from build123d import *

# Parameters (mm, degrees)
BOSS_EXTRUDE1_DEPTH     = 7
SKETCH2_R               = 5
CUT_EXTRUDE1_DEPTH      = 7
LPATTERN1_COUNT         = 7
LPATTERN1_PITCH         = 30
SKETCH6_R               = 5
CUT_EXTRUDE2_DEPTH      = 10
BOSS_EXTRUDE2_DEPTH     = 21
CUT_EXTRUDE3_DEPTH      = 21
CUT_EXTRUDE4_REACH      = 220.014
SKETCH9_R               = 1.5
CUT_EXTRUDE5_REACH      = 220.771
SKETCH10_W              = 5.271518542
SKETCH10_H              = 23.219312301
BOSS_EXTRUDE3_DEPTH     = 14
CUT_EXTRUDE6_DEPTH      = 1
CUT_EXTRUDE6_DEPTH_BACK = 22
SKETCH12_W              = 22.7
SKETCH12_H              = 12.3
CUT_EXTRUDE7_DEPTH      = 7
CUT_EXTRUDE7_DEPTH_BACK = 7
SKETCH13_R              = 1
CUT_EXTRUDE8_REACH      = 184.393
SKETCH14_W              = 12
SKETCH14_H              = 10
CUT_EXTRUDE9_REACH      = 220.014
SKETCH15_R              = 2.5


with BuildPart() as part:
    # Sketch1 → Boss-Extrude1 (new body)
    with BuildSketch(Plane.XY):
        with BuildLine():
            Line((-200, 0), (50, 0))
            ThreePointArc((50, 0), (65, -15), (50, -30))
            Line((50, -30), (-200, -30))
            ThreePointArc((-200, -30), (-215, -15), (-200, 0))
        make_face()
    extrude(amount=BOSS_EXTRUDE1_DEPTH)

    # Sketch2 → Cut-Extrude1 (cut)
    with BuildSketch(Plane.XY.offset(7)):
        with Locations((-185, -15)):
            Circle(SKETCH2_R)
    cut_extrude1 = extrude(amount=-CUT_EXTRUDE1_DEPTH, mode=Mode.SUBTRACT)

    # LPattern1: Cut-Extrude1 ×7
    with Locations(*[(i * LPATTERN1_PITCH, 0, 0) for i in range(1, LPATTERN1_COUNT)]):
        add(cut_extrude1, mode=Mode.SUBTRACT)

    # Sketch6 → Cut-Extrude2 (cut)
    with BuildSketch(Plane(origin=(0, 0, 0), x_dir=(-1, 0, 0), z_dir=(0, 0, -1))):
        with Locations((-50, -15)):
            Circle(SKETCH6_R)
    extrude(amount=-CUT_EXTRUDE2_DEPTH, mode=Mode.SUBTRACT)

    # Sketch7 → Boss-Extrude2 (add)
    with BuildSketch(Plane(origin=(0, 0, 0), x_dir=(0, 0, -1), z_dir=(1, 0, 0))):
        with BuildLine():
            Line((20.124409349, -8.046570755), (20.124409349, -21.391782887))
            ThreePointArc((20.124409349, -21.391782887), (10.062204675, -26.149434806), (0, -21.391782887))
            Line((0, -21.391782887), (0, -8.046570755))
            ThreePointArc((0, -8.046570755), (10.062204675, -2.930122505), (20.124409349, -8.046570755))
        make_face()
    extrude(amount=BOSS_EXTRUDE2_DEPTH)

    # Sketch8 → Cut-Extrude3 (cut)
    with BuildSketch(Plane(origin=(21, 0, 0), x_dir=(0, 0, -1), z_dir=(1, 0, 0))):
        with BuildLine():
            Line((0.343653188, -8.603738845), (0.343653188, -21.003738845))
            Line((0.343653188, -21.003738845), (3.251608919, -23.33010343))
            Line((3.251608919, -23.33010343), (6.11482687, -24.672236845))
            Line((6.11482687, -24.672236845), (10.141227113, -25.388041332))
            Line((10.141227113, -25.388041332), (14.122889575, -24.672236845))
            Line((14.122889575, -24.672236845), (17.165058648, -23.33010343))
            Line((17.165058648, -23.33010343), (19.670374355, -20.953281344))
            Line((19.670374355, -20.953281344), (19.670374355, -8.553281344))
            ThreePointArc((19.670374355, -8.553281344), (9.994377841, -3.738573545), (0.343653188, -8.603738845))
        make_face()
    extrude(amount=-CUT_EXTRUDE3_DEPTH, mode=Mode.SUBTRACT)

    # Sketch9 → Cut-Extrude4 (cut, up to next)
    with BuildSketch(Plane(origin=(0, 0, 0), x_dir=(-1, 0, 0), z_dir=(0, 0, -1)), mode=Mode.PRIVATE) as cut_extrude4_sk1:
        with Locations((-29.5, -6.25)):
            Circle(SKETCH9_R)
    cut_extrude4_tool1 = extrude(cut_extrude4_sk1.sketch, amount=-CUT_EXTRUDE4_REACH, mode=Mode.PRIVATE) & part.part
    # Sketch9 → Cut-Extrude4 (cut, up to next)
    with BuildSketch(Plane(origin=(0, 0, 0), x_dir=(-1, 0, 0), z_dir=(0, 0, -1)), mode=Mode.PRIVATE) as cut_extrude4_sk2:
        with Locations((-29.5, -23.75)):
            Circle(SKETCH9_R)
    cut_extrude4_tool2 = extrude(cut_extrude4_sk2.sketch, amount=-CUT_EXTRUDE4_REACH, mode=Mode.PRIVATE) & part.part
    add(cut_extrude4_tool1.solids().sort_by_distance((29.5, -6.25, 0))[0], mode=Mode.SUBTRACT)
    add(cut_extrude4_tool2.solids().sort_by_distance((29.5, -23.75, 0))[0], mode=Mode.SUBTRACT)

    # Cut-Extrude5: up to this face of the body (flat: up to its plane)
    cut_extrude5_end = Plane(part.part.faces().sort_by_distance((-78.33059512, -15.01080435, 0))[0])
    # Sketch10 → Cut-Extrude5 (cut, up to the picked face)
    with BuildSketch(Plane(origin=(0, 0, -20.124409349), x_dir=(-1, 0, 0), z_dir=(0, 0, -1)), mode=Mode.PRIVATE) as cut_extrude5_sk1:
        with Locations((-2.635759271, -14.539778656)):
            Rectangle(SKETCH10_W, SKETCH10_H)
    cut_extrude5_tool1 = split(extrude(cut_extrude5_sk1.sketch, amount=-CUT_EXTRUDE5_REACH, mode=Mode.PRIVATE), bisect_by=cut_extrude5_end, keep=Keep.BOTH, mode=Mode.PRIVATE)
    add(cut_extrude5_tool1.solids().sort_by(Axis((2.635759, -14.539779, -20.124409), (0, 0, 1)))[0], mode=Mode.SUBTRACT)

    # Sketch11 → Boss-Extrude3 (add)
    with BuildSketch(Plane(origin=(0, 0, 0), x_dir=(-1, 0, 0), z_dir=(0, 0, -1))):
        Polygon((60.097644306, -6.420008597), (60.097644306, -23.913431972), (36.21993437, -23.913431972), (36.21993437, -6.613282571), (31.020509523, -6.613282571), (31.020509523, -2.674883318), (65.276628567, -2.674883318), (65.276628567, -6.420008597), align=None)
        Polygon((193.975354243, -6.285954501), (193.975354243, -16.540829221), (170.097644306, -16.540829221), (170.097644306, -6.479228475), (164.898219459, -6.479228475), (164.898219459, -2.540829221), (199.154338504, -2.540829221), (199.154338504, -6.285954501), align=None)
    extrude(amount=BOSS_EXTRUDE3_DEPTH)

    # Sketch12 → Cut-Extrude6 (cut, two sides: drawn at the far end of the back side and taken through both)
    with BuildSketch(Plane(origin=(0, -2.674883318, 0), x_dir=(1, 0, 0), z_dir=(0, 1, 0)).offset(-CUT_EXTRUDE6_DEPTH_BACK)):
        with Locations((-48.226628567, 6.703751831)):
            Rectangle(SKETCH12_W, SKETCH12_H)
        with Locations((-182.104338504, 6.42306456)):
            Rectangle(SKETCH12_W, SKETCH12_H)
    extrude(amount=CUT_EXTRUDE6_DEPTH + CUT_EXTRUDE6_DEPTH_BACK, mode=Mode.SUBTRACT)

    # Sketch13 → Cut-Extrude7 (cut, two sides: drawn at the far end of the back side and taken through both)
    with BuildSketch(Plane(origin=(0, -2.674883318, 0), x_dir=(1, 0, 0), z_dir=(0, 1, 0)).offset(-CUT_EXTRUDE7_DEPTH_BACK)):
        with Locations(Location((-167.998219459, 8.19, 0), (0, 0, 90))):
            Circle(SKETCH13_R)
        with Locations(Location((-196.054338504, 8.19, 0), (0, 0, 90))):
            Circle(SKETCH13_R)
        with Locations(Location((-62.176628567, 8.19, 0), (0, 0, 90))):
            Circle(SKETCH13_R)
        with Locations(Location((-34.120509523, 8.19, 0), (0, 0, 90))):
            Circle(SKETCH13_R)
    extrude(amount=CUT_EXTRUDE7_DEPTH + CUT_EXTRUDE7_DEPTH_BACK, mode=Mode.SUBTRACT)

    # Cut-Extrude8: up to this face of the body (flat: up to its plane)
    cut_extrude8_end = Plane(part.part.faces().sort_by_distance((-193.975354243, -11.413391861, -7))[0])
    # Sketch14 → Cut-Extrude8 (cut, up to the picked face)
    with BuildSketch(Plane(origin=(-36.21993437, 0, 0), x_dir=(0, 0, -1), z_dir=(1, 0, 0)), mode=Mode.PRIVATE) as cut_extrude8_sk1:
        with Locations((8, -18.913431972)):
            Rectangle(SKETCH14_W, SKETCH14_H)
    cut_extrude8_tool1 = split(extrude(cut_extrude8_sk1.sketch, amount=-CUT_EXTRUDE8_REACH, mode=Mode.PRIVATE), bisect_by=cut_extrude8_end, keep=Keep.BOTH, mode=Mode.PRIVATE)
    add(cut_extrude8_tool1.solids().sort_by(Axis((-36.219934, -18.913432, -8), (-1, 0, 0)))[0], mode=Mode.SUBTRACT)

    # Sketch15 → Cut-Extrude9 (cut, up to next)
    with BuildSketch(Plane(origin=(0, 0, 0), x_dir=(1, 0, 0), z_dir=(0, 1, 0)), mode=Mode.PRIVATE) as cut_extrude9_sk1:
        with Locations(Location((-195.8, -3.5, 0), (0, 0, 180))):
            Circle(SKETCH15_R)
    cut_extrude9_tool1 = extrude(cut_extrude9_sk1.sketch, amount=-CUT_EXTRUDE9_REACH, mode=Mode.PRIVATE) & part.part
    # Sketch15 → Cut-Extrude9 (cut, up to next)
    with BuildSketch(Plane(origin=(0, 0, 0), x_dir=(1, 0, 0), z_dir=(0, 1, 0)), mode=Mode.PRIVATE) as cut_extrude9_sk2:
        with Locations(Location((45.8, -3.5, 0), (0, 0, 180))):
            Circle(SKETCH15_R)
    cut_extrude9_tool2 = extrude(cut_extrude9_sk2.sketch, amount=-CUT_EXTRUDE9_REACH, mode=Mode.PRIVATE) & part.part
    add(cut_extrude9_tool1.solids().sort_by_distance((-195.8, 0, 3.5))[0], mode=Mode.SUBTRACT)
    add(cut_extrude9_tool2.solids().sort_by_distance((45.8, 0, 3.5))[0], mode=Mode.SUBTRACT)


solid = part.part
Here's how the part is built. I have some questions about the finished solid (model axes, mm). A direction names the side the tool comes from. Coordinates: 2 decimals unless noted, no trailing zeros. Write each loop counter-clockwise with the first axis right and the second up, starting at its lowest first coordinate (ties: lowest second). Pieces come first, ordered by that corner, then holes.
Item 1: Will these pins go through, and if not, where does the flat tip stop? pin 1 (10 mm diameter, centred on y = -24.5, z = -8, fed in from -X); pin 2 (11.5 mm diameter, centred on x = -5, y = -15, fed in from -Z); pin 3 (0.6 mm diameter, centred on x = -184, z = -0.5, fed in from -Y).
Item 2: If I drill on line 1 (Y direction, x = 29.5, z = 3); line 2 (X direction, y = -5, z = -4.25); line 3 (X direction, y = -8, z = -10.5), over which ranges is the centre line in solid material (lowest first)?
Item 3: If we mould it in two halves opening along X, with no side actions, what happens to faces 4 (the flat face through (-73, -15, 7)), 5 (the cylindrical face through (43.49, -14.79, 2.54)), 6 (the cylindrical face through (65, -15, 3))? For each: +X half, -X half, draft (parallel to the pull), parting line (faces both ways), or undercut.
Item 4: I want a section at B-B on x = 10.5. Write out the boundary of the cut face in (y, z).
Item 5: I want a section at A-A on x = -125. Write out the boundary of the cut face in (y, z), and give its area (3 significant figures).
Item 6: On a 3-axis mill with a long thin cutter (end or side, diameter ignored), from which of +Z, -Z, +X, -X, +Y, -Y can I reach the whole of each face in a straight line? I mean faces 1 (the cylindrical face through (-189, -18, 4)), 2 (the flat face through (-178, -2.541, -13)), 3 (the flat face through (13, -15, -0.344)). Say none if no direction works.
Findings below:
1. pin 1: stops at x = 5.27
1. pin 2: stops at z = 0
1. pin 3: stops at y = -16.54
2. line 1: y = -30 to -25.25, -22.25 to -7.75, -4.75 to 0
2. line 2: x = -199.15 to -193.45, -170.75 to -164.9, -65.28 to -59.58, -36.88 to -31.02, 5.27 to 21
2. line 3: x = -193.98 to -193.45, -170.75 to -170.1, -60.1 to -59.58, -36.88 to -36.22
3. face 4: draft
3. face 5: undercut
3. face 6: +X half
4. outline: (-30, 0) - (-21.39, 0) arc R13.02 ccw to (-21.39, -20.12) - (-8.05, -20.12) arc R12.45 ccw to (-8.05, 0) - (0, 0) - (0, 7) - (-30, 7) - close; hole (-25.39, -10.14) - (-24.67, -14.12) - (-23.33, -17.17) - (-20.95, -19.67) - (-8.55, -19.67) arc R12.07 ccw to (-8.6, -0.34) - (-21, -0.34) - (-23.33, -3.25) - (-24.67, -6.11) - close
5. outline: (-30, 0) - (-20, 0) - (-20, 7) - (-30, 7) - close; (-10, 0) - (0, 0) - (0, 7) - (-10, 7) - close
5. area: 140 mm2
6. face 1: +Z
6. face 2: -Z, +X, -X, +Y
6. face 3: +X
